Could you check a few things on this model? Use its own coordinates, in mm. A direction names the side the tool comes from. Give positions to 0.01 mm unless a question says otherwise; leave off trailing zeros. Write each loop counter-clockwise with the first axis right and the second up, starting at its lowest first coordinate (ties: lowest second). Pieces come first, ordered by that corner, then holes. Notation, with made-up numbers: (-3, 42.5) - (10, 42.5) arc R19 cw to (10, 49.5) - close; hole circle Ø2 at (55.5, -35). An arc over 180 degrees is marked (long way). Write item = value, one per line.
from build123d import *

# Parameters (mm, degrees)
F0_R     = 4
F1_DEPTH = 25
F5_DEPTH = 4


with BuildPart() as f1:
    # F0 (on Front) → F1 (new body)
    with BuildSketch(Plane.XZ):
        Circle(F0_R)
    extrude(amount=F1_DEPTH)

    # F2 (on Right) → F3 (revolve)
    with BuildSketch(Plane.YZ):
        with BuildLine():
            Line((0, 7), (0, 0))
            Line((0, 0), (4.4, 0))
            Line((4.4, 0), (4.4, 2.5))
            Line((4.4, 2.5), (4.4, 3.5))
            ThreePointArc((4.4, 3.5), (2.811139, 6.018288), (0, 7))
        make_face()
    revolve(axis=Axis((0, 0, 0), (0, -1, 0)))

    # F4 (on face) → F5 (cut)
    with BuildSketch(Plane(origin=(0, 4.4, 0), x_dir=(-1, 0, 0), z_dir=(0, 1, 0))):
        Polygon((-2.5, 1.443376), (-2.5, -1.443376), (0, -2.886751), (2.5, -1.443376), (2.5, 1.443376), (0, 2.886751), align=None)
    extrude(amount=-F5_DEPTH, mode=Mode.SUBTRACT)


solid = f1.part
1. Thinking about a two-plate mould opening in Z: for faces 1 (the face through (2, 4.4, 2)), 2 (the face through (1.267, 2.428, -2.155)), 3 (the face through (-0.867, -12.325, -3.905)), which applies, pulls with the +Z half, pulls with the -Z half, needs draft (parallel to the pull), parting line crosses it, or undercut?
Filled sheet:
face_1 = needs draft
face_2 = undercut
face_3 = parting line crosses it
2. For pin 1 (2.5 mm diameter, centred on y = 2.5, z = 0.5, fed in from -X); pin 2 (3 mm diameter, centred on y = -20, z = -0.5, fed in from +X); pin 3 (2 mm diameter, centred on x = -2, y = -11.5, fed in from -Z), each with a flat end and sliding along its axis, tell me the tip position at first contact or that it passes through.
Filled sheet:
pin_1 = -6.81
pin_2 = 4
pin_3 = -3.87
3. I need wall thicknesses on line 1 (Y direction, x = -1.5, z = -1.75); line 2 (Z direction, x = 1.25, y = 2.25); line 3 (Z direction, x = 0.5, y = 0.5). Which ranges of each line are inside material? Lowest first, please.
Filled sheet:
line_1 = -25 to 0.4
line_2 = -6.28 to -2.17, 2.17 to 6.28
line_3 = -6.95 to -2.6, 2.6 to 6.95
4. If we section it at A-A, the plane y = -15.5: Please give me the cut outline in (x, z).
Filled sheet:
outline = circle Ø8 at (0, 0)
5. Which directions (+Z, -Z, +X, -X, +Y, -Y) give clear straight access to the entire face, cutting with the end or side of a thin tool? Please do faces 4 (the face through (3, 0, 3)), 5 (the face through (0, -25, 0)), 6 (the face through (-1.233, 2.428, -2.175)).
Filled sheet:
face_4 = -Y
face_5 = +Z, -Z, +X, -X, -Y
face_6 = +Y
